```python
from build123d import *


with BuildPart() as part:
    # Táhnout po křivce1: sweep along a path in Skica1
    with BuildLine(Plane.XY) as t_hnout_po_k_ivce1_path:
        Line((0, 0), (0, 60))
        ThreePointArc((0, 60), (1.464466094, 63.535533906), (5, 65))
        Line((5, 65), (20, 65))
    # Skica2 → Táhnout po křivce1 (sweep)
    with BuildSketch(Plane(origin=(0, 0, 0), x_dir=(1, 0, 0), z_dir=(0, 1, 0))):
        Polygon((1.5, 0.866025404), (0, 1.732050808), (-1.5, 0.866025404), (-1.5, -0.866025404), (0, -1.732050808), (1.5, -0.866025404), align=None)
    sweep(path=t_hnout_po_k_ivce1_path.line)


solid = part.part
```
Input: part model. Units: mm. Frame: model coordinates. A direction names the side the tool comes from. Coordinates: 2 decimals unless noted, no trailing zeros. Loops run counter-clockwise (first coordinate to the right, second up) from the corner with the lowest first, then second, coordinate; pieces in that order, holes last. Notation, with made-up numbers: M 12.25,43.5 L 25.25,43.5 A28 cw 25.25,78.5 Z; hole C 29.5,30.25 d6. An arc over 180 degrees is marked long. Answer in a Markdown table with one row per item.
1. Section B-B, the plane y = 22.5. Output: boundary loops of the cut face in (x, z), then the cut area to 3 significant figures.
Response:
| item | result |
|---|---|
| outline | M -1.5,-0.87 L 0,-1.73 L 1.5,-0.87 L 1.5,0.87 L 0,1.73 L -1.5,0.87 Z |
| area | 7.79 mm2 |
2. Section C-C, the plane x = 8.5. Output: boundary loops of the cut face in (y, z).
Response:
| item | result |
|---|---|
| outline | M 63.5,-0.87 L 65,-1.73 L 66.5,-0.87 L 66.5,0.87 L 65,1.73 L 63.5,0.87 Z |
3. First-contact query: pin 1 (1.4 mm diameter, centred on x = 10.5, z = -0.5, fed in from -Y); pin 2 (0.5 mm diameter, centred on y = 24.5, z = 0, fed in from +X); pin 3 (1.5 mm diameter, centred on x = 1.5, z = 0.5, fed in from +Y). Flat tips, straight axial feed; report the tip coordinate or a pass-through.
Response:
| item | result |
|---|---|
| pin 1 | stops at y = 63.5 |
| pin 2 | stops at x = 1.5 |
| pin 3 | stops at y = 65.89 |
4. Section A-A, the plane z = 0.3. Output: boundary loops of the cut face in (x, y).
Response:
| item | result |
|---|---|
| outline | M -1.5,0 L 1.5,0 L 1.5,60 A3.5 cw 5,63.5 L 20,63.5 L 20,66.5 L 5,66.5 A6.5 ccw -1.5,60 Z |
5. Material intervals for line 1 (X direction, y = 31, z = -0.15); line 2 (Y direction, x = 8, z = 0.25); line 3 (X direction, y = 8.5, z = 1.3), sorted ascending.
Response:
| item | result |
|---|---|
| line 1 | x = -1.5 to 1.5 |
| line 2 | y = 63.5 to 66.5 |
| line 3 | x = -0.75 to 0.75 |
6. Reachability of faces 1 (the flat face through (13, 63.5, 0)), 2 (the flat face through (12.605, 64.26, 1.305)), 3 (the flat face through (0.76, 30.42, -1.293)) from +Z, -Z, +X, -X, +Y, -Y: full face, straight path, thin tool, end or side. Return the list, or none.
Response:
| item | result |
|---|---|
| face 1 | +Z, -Z, +X, -Y |
| face 2 | +Z, +X, -Y |
| face 3 | -Z, +X, -Y |
